Autodesk Inventor part; units mm, degrees
ref_plane "YZ Plane" through (0, 0, 0) normal (1, 0, 0) x (0, 1, 0)
ref_plane "XZ Plane" through (0, 0, 0) normal (0, 1, 0) x (-1, 0, 0)
ref_plane "XY Plane" through (0, 0, 0) normal (0, 0, 1) x (1, 0, 0)
sketch "Base" plane through (0, 0, 0) normal (0, 0, 1) x (1, 0, 0)
  arc A0 (-53.9833, -2.5) -> (-40.2726, -6.1797) centre (-46.5, -2) ccw
  line L0 (-6.0829, -4.3873) -> (-40.2726, -6.1797)
  arc A1 (-6.0829, -4.3873) -> (6.3177, -4.0419) centre (0, 0) ccw
  line L1 (60.0086, 15.5) -> (6.3177, -4.0419)
  circle A2 centre (52, 20.5) radius 1.5 construction
  circle A3 centre (28, 20.5) radius 1.5 construction
  line L2 (57.0167, 27.5) -> (60.0086, 15.5)
  line L3 (57.0167, 27.5) -> (-53.9833, 27.5)
  line L4 (-53.9833, -2.5) -> (-53.9833, 27.5)
  line L5 (52, 20.5) -> (28, 20.5) construction
  dimension "d3" = 24
  dimension "d4" = 3
  dimension "d7" = 104
  dimension "d16" = 20
  dimension "d17" = 111
  dimension "d19" = 30
  dimension "d22" = 86.999
  dimension "d25" = 28
  dimension "d26" = 7.5
  dimension "d31" = 27.5
  dimension "d32" = 12
  dimension "d45" = 46.5
  dimension "d46" = 2
  dimension "d47" = 4.5
  dimension "d64" = 7
extrude "BaseFeature" add sketch "Base" along normal blind 4
fillet "EndFilletsFeature" radius 1 2 edges at (60.0086, 15.5, 2) (57.0167, 27.5, 2)
sketch "BaseMountHoles" plane through (0, 0, 0) normal (0, 0, -1) x (-1, 0, 0)
  arc A0 (40.2726, -6.1797) -> (53.9833, -2.5) centre (46.5, -2) ccw
  point P0 (0, 0)
hole "BaseMountHolesFeature" at (-46.5, -2, 0) at (0, 0, 0) direction (0, 0, 1) diameter 6 end through all
sketch "CuffMountHoles" plane through (0, 0, 0) normal (0, 0, -1) x (-1, 0, 0)
  circle A0 centre (-52, 20.5) radius 1.5 construction
  circle A1 centre (-28, 20.5) radius 1.5 construction
  point P0 (0, 0)
hole "CuffMountHolesFeature" at (52, 20.5, 0) at (28, 20.5, 0) direction (0, 0, 1) diameter 3 end through all
sketch "ExternalAssemblyGeometry" plane through (0, 0, 4) normal (0, 0, 1) x (1, 0, 0)
  circle A0 centre (-4.2211, 14.5) radius 2.4585 construction
  circle A1 centre (-12.2211, 14.5) radius 2.4585 construction
  circle A2 centre (-33.6105, 14.5) radius 2.4585 construction
  circle A3 centre (-55, 14.5) radius 2.4585 construction
  line L0 (16.9953, 21.5) -> (-152.0047, 21.5) construction
  line L1 (-55, 14.5) -> (12, 14.5) construction
  circle A4 centre (-55, 14.5) radius 7
  line L2 (-53.9833, 27.5) -> (56.2354, 27.5)
  line L3 (-53.9833, -2.5) -> (-53.9833, 27.5)
  dimension "d57" = 67
  dimension "d72" = 14
  dimension "d73" = 6
  dimension "d74" = 169
  dimension "d75" = 4.917
  dimension "d76" = 8
  dimension "d77" = 1.0167
  dimension "d78" = 21.3895
  dimension "d79" = 21.3895
  dimension "d80" = 70.9786
extrude "MountRailEndFeature" add sketch "ExternalAssemblyGeometry" against normal up to surface (4 mm away)
sketch "MountRail" plane through (0, 0, 0) normal (0, 0, -1) x (-1, 0, 0)
  line L0 (55, 14.5) -> (-12, 14.5) construction
  circle A0 centre (55, 14.5) radius 2.4585 construction
  circle A1 centre (-12, 14.5) radius 2.4585
  circle A2 centre (55, 14.5) radius 2.4585
  line L1 (55, 12.0415) -> (-12, 12.0415)
  line L2 (55, 16.9585) -> (-12, 16.9585)
  point P0 (0, 0)
extrude "MountRailFeature" cut sketch "MountRail" against normal through all
sketch "TopAngleCut" plane through (0, 0, 0) normal (0, 0, -1) x (-1, 0, 0)
  line L0 (53.9833, 27.5) -> (-56.2354, 27.5) construction
  line L1 (-22.2354, 27.5) -> (-18.7284, 21.4258)
  line L2 (53.9833, 21.4258) -> (-18.7284, 21.4258)
  line L3 (-22.2354, 27.5) -> (53.9833, 27.5)
  line L4 (53.9833, 21.4258) -> (53.9833, 27.5)
  line L5 (53.9833, 21.4258) -> (53.9833, 27.5)
  point P0 (0, 0)
  point P1 (-57.0167, 27.5)
  dimension "d65" = 120
  dimension "d66" = 34
extrude "TopAngleCutFeature" cut sketch "TopAngleCut" against normal through all
fillet "TopAngleCutFilletsFeature" radius 1 2 edges at (22.2354, 27.5, 2) (18.7284, 21.4258, 2)
fillet "BodyFilletFeature" radius 1 2 edges at (-53.9833, 21.4258, 2) (-53.9833, 7.5742, 2)
properties part number "ForearmLeftEnd"
Geometry check sheet. Reference: the model listing, model coordinates, mm. A direction names the side the tool comes from. Round coordinates to 2 decimals unless told otherwise and drop trailing zeros. Write each loop counter-clockwise with the first axis right and the second up, starting at its lowest first coordinate (ties: lowest second). Pieces come first, ordered by that corner, then holes.
Item 1: Mould release check, pull along Y, two halves, no side actions. Record for faces 1 (the face through (-2, 9, 4)), 2 (the face through (20.502, 24.498, 1.972)), 3 (the face through (-22, 16.958, 2)), 4 (the face through (-48.318, -9.276, 1.972)): +Y half, -Y half, draft (parallel to the pull), parting line (faces both ways), or undercut.
Determined:
face 1: draft
face 2: +Y half
face 3: undercut
face 4: -Y half
Item 2: Material ranges on line 1 along Y through (x, z) = (-46.5, 1.1); line 2 along Y through (x, z) = (0, 2.45); line 3 along X through (y, z) = (20.5, 3.05), recorded low to high.
Determined:
line 1: y = -9.5 to -5, 1 to 12.04, 16.96 to 21.43
line 2: y = -7.5 to -3, 3 to 12.04, 16.96 to 21.43
line 3: x = -58.61 to 26.5, 29.5 to 50.5, 53.5 to 58.76
Item 3: Section check A-A (x = -11.5). Record the boundary of the cut face in (y, z).
Determined:
outline: (-4.67, 0) - (12.04, 0) - (12.04, 4) - (-4.67, 4) - close; (16.96, 0) - (21.43, 0) - (21.43, 4) - (16.96, 4) - close
Item 4: Section check C-C (x = 52). Record the boundary of the cut face in (y, z).
Determined:
outline: (12.59, 0) - (19, 0) - (19, 4) - (12.59, 4) - close; (22, 0) - (27.5, 0) - (27.5, 4) - (22, 4) - close
Item 5: Access from +Z, -Z, +X, -X, +Y, -Y to the whole of each face (thin tool, end or side, straight path). Record for faces 5 (the face through (-53.983, 2, 2)), 6 (the face through (-22.94, -5.27, 1.97)), 7 (the face through (-57.458, 14.446, 1.972)), 8 (the face through (40, 27.5, 2)).
Determined:
face 5: +Z, -Z, -X, -Y
face 6: +Z, -Z, -Y
face 7: +Z, -Z
face 8: +Z, -Z, +X, -X, +Y
Item 6: Section check B-B (z = 3.15). Record the boundary of the cut face in (x, y).
Determined:
outline: (-54.99, 7.5) arc R1 cw to (-53.98, 6.5) - (-53.98, -2.5) arc R7.5 ccw to (-40.27, -6.18) - (-6.08, -4.39) arc R7.5 ccw to (6.32, -4.04) - (59.16, 15.19) arc R1 ccw to (59.79, 16.37) - (57.21, 26.74) arc R1 ccw to (56.24, 27.5) - (22.81, 27.5) arc R1 ccw to (21.95, 27) - (19.02, 21.93) arc R1 cw to (18.15, 21.43) - (-53.91, 21.43) arc R1 cw to (-54.05, 21.44) arc R7 ccw (long way) to start; hole (-55, 12.04) - (12, 12.04) arc R2.46 ccw to (12, 16.96) - (-55, 16.96) arc R2.46 ccw to start; hole circle Ø6 at (-46.5, -2); hole circle Ø6 at (0, 0); hole circle Ø3 at (28, 20.5); hole circle Ø3 at (52, 20.5)
Item 7: Go/stop test with flat-tipped pins: pin 1 Ø2 at (x, z) = (-33, 1.5) entering from -Y; pin 2 Ø1 at (x, z) = (42.5, 1) entering from -Y; pin 3 Ø1.5 at (x, z) = (-27.5, 2) entering from -Y. Record where each tip stops, or that it passes through.
Determined:
pin 1: stops at y = -5.85
pin 2: stops at y = 8.95
pin 3: stops at y = -5.55
Item 8: Section check D-D (y = 24). Record the boundary of the cut face in (x, z), plus the area to 3 significant figures.
Determined:
outline: (20.21, 0) - (57.89, 0) - (57.89, 4) - (20.21, 4) - close
area: 151 mm2
